The listing builds one solid part. Answer for the finished solid, in the listing's coordinates (mm). Coordinates: 2 decimals unless noted, no trailing zeros. Write each loop counter-clockwise with the first axis right and the second up, starting at its lowest first coordinate (ties: lowest second). Pieces come first, ordered by that corner, then holes.
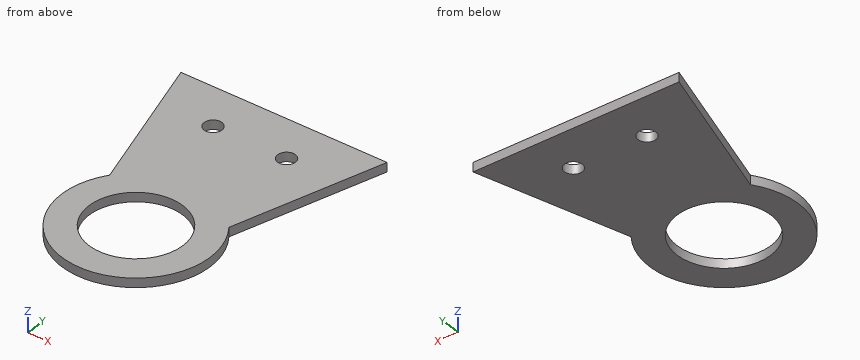
from build123d import *

# Parameters (mm, degrees)
SKETCH1_W               = 70
SKETCH1_H               = 100
SKETCH1_R               = 15.8115
SKETCH1_R_2             = 3
BOSS_EXTRUDE1_DEPTH     = 3.1
CUT_EXTRUDE1_DEPTH      = 1
CUT_EXTRUDE1_DEPTH_BACK = 4.1


with BuildPart() as part:
    # Sketch1 → Boss-Extrude1 (new body)
    with BuildSketch(Plane.XY):
        with Locations((0, 15)):
            Rectangle(SKETCH1_W, SKETCH1_H)
        Circle(SKETCH1_R, mode=Mode.SUBTRACT)
        with Locations((-12.5, 50)):
            Circle(SKETCH1_R_2, mode=Mode.SUBTRACT)
        with Locations((12.5, 50)):
            Circle(SKETCH1_R_2, mode=Mode.SUBTRACT)
    extrude(amount=BOSS_EXTRUDE1_DEPTH)

    # Sketch2 → Cut-Extrude1 (cut, two sides)
    with BuildSketch(Plane.XY.offset(3.1)) as cut_extrude1_sk:
        with BuildLine():
            Line((-106.300801708, 308.923795317), (-35, 65))
            Line((-35, 65), (-20.275240011, 14.625821089))
            ThreePointArc((-20.275240011, 14.625821089), (0, -25), (20.275240011, 14.625821089))
            Line((20.275240011, 14.625821089), (35, 65))
            Line((35, 65), (106.300801708, 308.923795317))
            Line((106.300801708, 308.923795317), (106.300801708, -199.338429312))
            Line((106.300801708, -199.338429312), (-106.300801708, -199.338429312))
            Line((-106.300801708, -199.338429312), (-106.300801708, 308.923795317))
        make_face()
    extrude(amount=CUT_EXTRUDE1_DEPTH, mode=Mode.SUBTRACT)
    extrude(cut_extrude1_sk.sketch, amount=-CUT_EXTRUDE1_DEPTH_BACK, mode=Mode.SUBTRACT)


solid = part.part
1. Find the intervals of material crossed by L1, parallel to Y at x = -12.5, z = 1.3; L2, parallel to Y at x = 0, z = 2.35; L3, parallel to Y at x = -10.5, z = 2.95, in increasing order.
Results found:
L1: y = -21.65 to -9.68, 9.68 to 47, 53 to 65
L2: y = -25 to -15.81, 15.81 to 65
L3: y = -22.69 to -11.82, 11.82 to 47.76, 52.24 to 65
2. Section B-B on y = 11.5 is taken. Give the vertices of the cut face in (x, z).
Results found:
outline: (-22.2, 0) - (-10.85, 0) - (-10.85, 3.1) - (-22.2, 3.1) - close; (10.85, 0) - (22.2, 0) - (22.2, 3.1) - (10.85, 3.1) - close
3. Flat-ended cylindrical pins translate along their axes: P1, Ø4, axis at x = -26.5, y = -4.5, coming from the -Z side; P2, Ø1, axis at y = 47, z = 2, coming from the +X side. Find the tip coordinate at first contact, or state that the pin passes through.
Results found:
P1: stops at z = 0
P2: stops at x = 29.88
4. Section D-D on x = -12.5 is taken. Give the vertices of the cut face in (y, z), then the cut area to 3 significant figures.
Results found:
outline: (-21.65, 0) - (-9.68, 0) - (-9.68, 3.1) - (-21.65, 3.1) - close; (9.68, 0) - (47, 0) - (47, 3.1) - (9.68, 3.1) - close; (53, 0) - (65, 0) - (65, 3.1) - (53, 3.1) - close
area: 190 mm2
5. Section C-C on z = 2.1 is taken. Give the vertices of the cut face in (x, y), then the cut area to 3 significant figures.
Results found:
outline: (-35, 65) - (-20.28, 14.63) arc R25 ccw (long way) to (20.28, 14.63) - (35, 65) - close; hole circle Ø31.62 at (0, 0); hole circle Ø6 at (-12.5, 50); hole circle Ø6 at (12.5, 50)
area: 3,610 mm2
6. Section A-A on x = 0 is taken. Give the vertices of the cut face in (y, z).
Results found:
outline: (-25, 0) - (-15.81, 0) - (-15.81, 3.1) - (-25, 3.1) - close; (15.81, 0) - (65, 0) - (65, 3.1) - (15.81, 3.1) - close
